```python
from build123d import *

# Parameters (mm, degrees)
F0_W         = 88
F0_H         = 3
F1_DEPTH     = 30
F2_R         = 3
F3_T1_DEPTH  = 142
F3_T3_DEPTH  = 90
F3_T5_DEPTH  = 180
F3_T7_DEPTH  = 29
F3_T10_ANGLE = 90
F3_T12_ANGLE = 90
F4_W         = 7.4076932669
F4_H         = 3.6282110959
F4_H_2       = 3.7070848048
F5_DEPTH     = 3
F6_W         = 11.1425933428
F6_H         = 19.764843164
F6_W_2       = 10.4046501219
F6_H_2       = 19.7511005681
F6_W_3       = 9.5925889909
F6_W_4       = 10.5412900448
F6_W_5       = 10.9199807048
F6_W_6       = 10.6662213802
F6_W_7       = 10.4241892695
F7_DEPTH     = 3
F8_R         = 1


# Not quite as in the source:
# - a fillet or chamfer that OpenCascade refuses, or shapes differently, is made with other operations: its cross-section is extruded or revolved along the edge and cut away or added


with BuildPart() as f1:
    # F0 (on Top) → F1 (new body)
    with BuildSketch(Plane.XY):
        Polygon((3, 0), (0, 0), (0, -140), (0, -143), (0, -170), (3, -170), (3, -140), align=None)
        with Locations((-44, -141.5)):
            Rectangle(F0_W, F0_H)
    extrude(amount=F1_DEPTH)

    # F2
    f2_edges = [f1.edges().sort_by_distance(p)[0] for p in [
        (0, -140, 15),
        (0, -143, 15),
    ]]
    fillet(f2_edges, radius=F2_R)

    # F3: fillet of radius 2 on 3 edges, made by hand

    # F3_s2 → F3_t1 (cut)
    with BuildSketch(Plane.XZ.offset(-5)):
        with BuildLine():
            ThreePointArc((0, 28), (0.5857864376, 29.4142135624), (2, 30))
            Line((2, 30), (0, 30))
            Line((0, 30), (0, 28))
        make_face()
    extrude(amount=F3_T1_DEPTH, mode=Mode.SUBTRACT)

    # F3_s4 → F3_t3 (cut)
    with BuildSketch(Plane.YZ.offset(-93)):
        with BuildLine():
            ThreePointArc((-141, 30), (-142.4142135624, 29.4142135624), (-143, 28))
            Line((-143, 28), (-143, 30))
            Line((-143, 30), (-141, 30))
        make_face()
        with BuildLine():
            ThreePointArc((-142, 30), (-140.5857864376, 29.4142135624), (-140, 28))
            Line((-140, 28), (-140, 30))
            Line((-140, 30), (-142, 30))
        make_face()
    extrude(amount=F3_T3_DEPTH, mode=Mode.SUBTRACT)

    # F3_s6 → F3_t5 (cut)
    with BuildSketch(Plane.XZ.offset(-5)):
        with BuildLine():
            ThreePointArc((1, 30), (2.4142135624, 29.4142135624), (3, 28))
            Line((3, 28), (3, 30))
            Line((3, 30), (1, 30))
        make_face()
    extrude(amount=F3_T5_DEPTH, mode=Mode.SUBTRACT)

    # F3_s8 → F3_t7 (cut)
    with BuildSketch(Plane.XZ.offset(146)):
        with BuildLine():
            ThreePointArc((2, 30), (0.5857864376, 29.4142135624), (0, 28))
            Line((0, 28), (0, 30))
            Line((0, 30), (2, 30))
        make_face()
    extrude(amount=F3_T7_DEPTH, mode=Mode.SUBTRACT)

    # F3_s9 → F3_t10 (revolve, cut)
    with BuildSketch(Plane.YZ.offset(-3)):
        with BuildLine():
            ThreePointArc((-141, 30), (-142.4142135624, 29.4142135624), (-143, 28))
            Line((-143, 28), (-143, 30))
            Line((-143, 30), (-141, 30))
        make_face()
    revolve(axis=Axis((-3, -146, 30), (0, 0, -1)), revolution_arc=F3_T10_ANGLE, mode=Mode.SUBTRACT)

    # F3_s11 → F3_t12 (revolve, cut)
    with BuildSketch(Plane.XZ.offset(137)):
        with BuildLine():
            ThreePointArc((0, 28), (0.5857864376, 29.4142135624), (2, 30))
            Line((2, 30), (0, 30))
            Line((0, 30), (0, 28))
        make_face()
    revolve(axis=Axis((-3, -137, 30), (0, 0, -1)), revolution_arc=F3_T12_ANGLE, mode=Mode.SUBTRACT)

    # F4 (on face) → F5 (cut)
    with BuildSketch(Plane(origin=(0, 0, 0), x_dir=(0, -1, 0), z_dir=(-1, 0, 0))):
        with Locations((166.2961533666, 22.8808587417)):
            Rectangle(F4_W, F4_H)
        with Locations((166.2961533666, 9.8271891475)):
            Rectangle(F4_W, F4_H_2)
    extrude(amount=-F5_DEPTH, mode=Mode.SUBTRACT)

    # F6 (on face) → F7 (cut)
    with BuildSketch(Plane(origin=(0, 0, 0), x_dir=(0, -1, 0), z_dir=(-1, 0, 0))):
        with Locations((12.6331185456, 13.5222995887)):
            Rectangle(F6_W, F6_H)
        with Locations((32.683422789, 13.5154282907)):
            Rectangle(F6_W_2, F6_H_2)
        with Locations((51.4230821282, 13.5154282907)):
            Rectangle(F6_W_3, F6_H_2)
        with Locations((68.6303824186, 13.5154282907)):
            Rectangle(F6_W_4, F6_H_2)
        with Locations((85.6932289898, 13.5154282907)):
            Rectangle(F6_W_5, F6_H_2)
        with Locations((103.2284647226, 13.5154282907)):
            Rectangle(F6_W_6, F6_H_2)
        with Locations((120.2503331006, 13.5154282907)):
            Rectangle(F6_W_7, F6_H_2)
    extrude(amount=-F7_DEPTH, mode=Mode.SUBTRACT)

    # F8
    f8_edges = [f1.edges().sort_by_distance(p)[0] for p in [
        (1.5, -7.061822, 23.404721),
        (1.5, -27.481098, 23.390979),
        (1.5, -46.626788, 23.390979),
        (1.5, -63.359737, 23.390979),
        (1.5, -80.233239, 23.390979),
        (1.5, -97.895354, 23.390979),
        (1.5, -115.038238, 23.390979),
        (1.5, -7.061822, 3.639878),
        (1.5, -27.481098, 3.639878),
        (1.5, -46.626788, 3.639878),
        (1.5, -63.359737, 3.639878),
        (1.5, -80.233239, 3.639878),
        (1.5, -97.895354, 3.639878),
        (1.5, -115.038238, 3.639878),
        (1.5, -125.462428, 23.390979),
        (1.5, -108.561575, 23.390979),
        (1.5, -91.153219, 23.390979),
        (1.5, -73.901027, 23.390979),
        (1.5, -56.219377, 23.390979),
        (1.5, -37.885748, 23.390979),
        (1.5, -18.204415, 23.404721),
        (1.5, -18.204415, 3.639878),
        (1.5, -37.885748, 3.639878),
        (1.5, -56.219377, 3.639878),
        (1.5, -73.901027, 3.639878),
        (1.5, -91.153219, 3.639878),
        (1.5, -108.561575, 3.639878),
        (1.5, -125.462428, 3.639878),
    ]]
    fillet(f8_edges, radius=F8_R)


solid = f1.part
```
Verification items for the finished model (mm, model axes). A direction names the side the tool comes from. Coordinates: 2 decimals unless noted, no trailing zeros. Order: outer loops, then holes, each group sorted by start corner. A loop starts at its lowest first (then second) coordinate and runs counter-clockwise, first axis right, second up. Notation, with made-up numbers: (-29, 89.5) -> (-3, 89.5) arc R24 cw to (-3, 127.5) -> close; hole circle Ø10 at (18, -12). An arc over 180 degrees is marked (long way). Put each result on its own line as item: value. Start each with the question number.
1) Cross-section at B-B (y = -113). Enter the section's corners in (x, z).
2) Cross-section at C-C (x = -67.5). Enter the section's corners in (y, z), plus the area to 3 significant figures.
3) Tool access check on faces 1 (the flat face through (1, -170, 4)), 2 (the flat face through (1, -46.627, 13)), 3 (the flat face through (1, -162.592, 23)). Record the directions out of +Z, -Z, +X, -X, +Y, -Y that give a thin tool (end or side, any length) a straight path to the whole face; none if there is none.
4) Material ranges on L1, parallel to Y at x = -32.5, z = 4; L2, parallel to X at y = -156, z = 3; L3, parallel to Z at x = -79, y = -142, recorded low to high.
5) Go/stop test with flat-tipped pins: pin 1 (1.5 mm diameter, centred on x = 1.5, y = -119, fed in from -Z); pin 2 (3.5 mm diameter, centred on x = 2, y = -11.5, fed in from +Z); pin 3 (1.5 mm diameter, centred on x = 1, z = 9.5, fed in from -Y); pin 4 (12 mm diameter, centred on y = -33.5, z = 7.5, fed in from -X). Record where each tip stops, or that it passes through.
6) Release check for a two-part mould opening along Z. For faces 4 (the flat face through (1, -51, 3.64)), 5 (the cylindrical face through (-0.86, -139.1, 14.2)) record: pulls with the +Z half, pulls with the -Z half, needs draft (parallel to the pull), parting line crosses it, or undercut.
7) Cross-section at A-A (z = 19). State how many separate pieces and enclosed holes the cut face has, plus the area to 3 significant figures.
Geometry check:
1. outline: (0, 0) -> (3, 0) -> (3, 28) arc R2 ccw to (1.5, 29.94) arc R2 ccw to (0, 28) -> close
2. outline: (-143, 0) -> (-140, 0) -> (-140, 28) arc R2 ccw to (-141.5, 29.94) arc R2 ccw to (-143, 28) -> close
2. area: 88.3 mm^2
3. face 1: +Z, -Z, +X, -X, -Y
3. face 2: +X, -X
3. face 3: +X, -X, -Y
4. L1: y = -143 to -140
4. L2: x = 0 to 3
4. L3: z = 0 to 29.73
5. pin 1: stops at z = 0
5. pin 2: stops at z = 29.94
5. pin 3: stops at y = -162.59
5. pin 4: stops at x = 0
6. face 4: undercut
6. face 5: needs draft
7. separate pieces: 8
7. enclosed holes: 0
7. area: 557 mm^2
